Build history of the part. All positions in model axes, mm. Face numbers are marked on the shaded views. A direction names the side the tool comes from. Round coordinates to 2 decimals unless told otherwise and drop trailing zeros. Write each loop counter-clockwise with the first axis right and the second up, starting at its lowest first coordinate (ties: lowest second). Pieces come first, ordered by that corner, then holes. Notation, with made-up numbers: (19.5, -17) -> (32.5, -17) arc R13 ccw to (32.5, -10) -> close; hole circle Ø2 at (79.25, 52). An arc over 180 degrees is marked (long way). Answer in a Markdown table with one row per item.
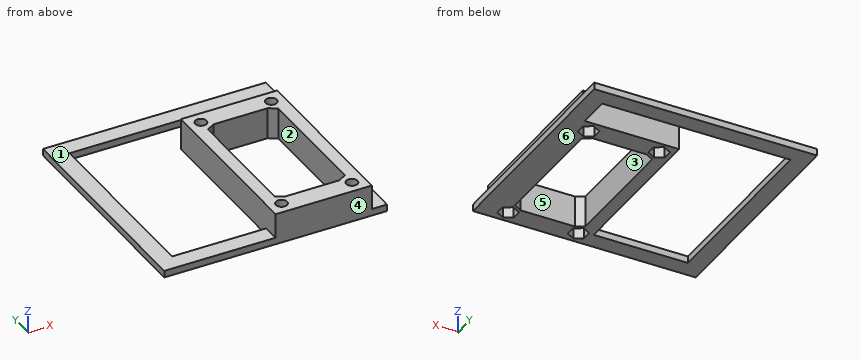
Autodesk Fusion 360 part; units mm, degrees
sketch "Sketch1" plane through (0, 0, 0) normal (0, 0, 1) x (1, 0, 0)
  line L0 (0, 0) -> (-65, 0)
  line L1 (-65, 0) -> (-65, 65)
  line L2 (-65, 65) -> (0, 65)
  line L3 (0, 65) -> (0, 0)
  line L4 (-32.5, 65) -> (-32.5, 0)
  line L5 (-28.75, 1) -> (-26.3684, 2.375)
  line L6 (-26.3684, 2.375) -> (-26.3684, 5.125)
  line L7 (-26.3684, 5.125) -> (-28.75, 6.5)
  line L8 (-28.75, 6.5) -> (-31.1316, 5.125)
  line L9 (-31.1316, 5.125) -> (-31.1316, 2.375)
  line L10 (-31.1316, 2.375) -> (-28.75, 1)
  line L11 (-28.75, 44.19) -> (-26.3684, 45.565)
  line L12 (-26.3684, 45.565) -> (-26.3684, 48.315)
  line L13 (-26.3684, 48.315) -> (-28.75, 49.69)
  line L14 (-28.75, 49.69) -> (-31.1316, 48.315)
  line L15 (-31.1316, 48.315) -> (-31.1316, 45.565)
  line L16 (-31.1316, 45.565) -> (-28.75, 44.19)
  line L17 (-28.75, 49.69) -> (-28.75, 50.69)
  line L18 (-28.75, 50.69) -> (-32.5, 50.69)
  line L19 (-28.75, 50.69) -> (0, 50.69)
  line L20 (-65, 0) -> (-60, 0)
  line L21 (-60, 0) -> (-60, 5)
  line L22 (-60, 5) -> (-65, 5)
  line L23 (-65, 5) -> (-65, 0)
  line L24 (-65, 65) -> (-60, 65)
  line L25 (-60, 65) -> (-60, 60)
  line L26 (-60, 60) -> (-65, 60)
  line L27 (-65, 60) -> (-65, 65)
  line L28 (0, 65) -> (-5, 65)
  line L29 (-5, 65) -> (-5, 60)
  line L30 (-5, 60) -> (0, 60)
  line L31 (0, 60) -> (0, 65)
  line L32 (-5, 60) -> (-60, 60)
  line L33 (-60, 60) -> (-60, 65)
  line L34 (-60, 65) -> (-5, 65)
  line L35 (-5, 65) -> (-5, 60)
  line L36 (-60, 60) -> (-65, 60)
  line L37 (-65, 60) -> (-65, 5)
  line L38 (-65, 5) -> (-60, 5)
  line L39 (-60, 5) -> (-60, 60)
  line L40 (-60, 0) -> (-32.5, 0)
  line L41 (-32.5, 0) -> (-32.5, 5)
  line L42 (-32.5, 5) -> (-60, 5)
  line L43 (-60, 5) -> (-60, 0)
  line L44 (-28.75, 6.5) -> (-28.75, 7.5)
  line L45 (-28.75, 7.5) -> (-26.3684, 6.125)
  line L46 (-28.75, 44.19) -> (-28.75, 43.19)
  line L47 (-3.75, 44.19) -> (-3.75, 43.19)
  line L48 (-26.3684, 44.565) -> (-28.75, 43.19)
  line L49 (-28.75, 7.5) -> (-28.75, 43.19)
  circle A0 centre (-28.75, 46.94) radius 1.65
  circle A1 centre (-28.75, 3.75) radius 1.65
  line L50 (-5, 60) -> (-5, 50.69)
  line L51 (-28.75, 46.94) -> (-8.2, 46.94)
  circle A2 centre (-8.2, 46.94) radius 1.65
  line L52 (-28.75, 3.75) -> (-8.2, 3.75)
  circle A3 centre (-8.2, 3.75) radius 1.65
  line L53 (-8.2, 1) -> (-5.8184, 2.375)
  line L54 (-5.8184, 2.375) -> (-5.8184, 5.125)
  line L55 (-5.8184, 5.125) -> (-8.2, 6.5)
  line L56 (-8.2, 6.5) -> (-10.5816, 5.125)
  line L57 (-10.5816, 5.125) -> (-10.5816, 2.375)
  line L58 (-10.5816, 2.375) -> (-8.2, 1)
  line L59 (-8.2, 44.19) -> (-5.8184, 45.565)
  line L60 (-5.8184, 45.565) -> (-5.8184, 48.315)
  line L61 (-5.8184, 48.315) -> (-8.2, 49.69)
  line L62 (-8.2, 49.69) -> (-10.5816, 48.315)
  line L63 (-10.5816, 48.315) -> (-10.5816, 45.565)
  line L64 (-10.5816, 45.565) -> (-8.2, 44.19)
  line L65 (-8.2, 44.19) -> (-8.2, 43.19)
  line L66 (-8.2, 43.19) -> (-10.5816, 44.565)
  line L67 (-10.5816, 44.565) -> (-26.3684, 44.565)
  line L68 (-8.2, 43.19) -> (-8.2, 7.5)
  line L69 (-8.2, 7.5) -> (-10.5816, 6.125)
  line L70 (-10.5816, 6.125) -> (-26.3684, 6.125)
  line L71 (-8.2, 25.345) -> (-4.45, 25.345)
  line L72 (-4.45, 25.345) -> (-4.45, 0)
  line L73 (-4.45, 25.345) -> (-4.45, 50.69)
  point P0 (-28.75, 3.75)
  point P1 (-28.75, 46.94)
  point P2 (-8.2, 3.75)
  point P3 (-8.2, 46.94)
  dimension "d1" = 65
  dimension "d2" = 65
  dimension "d10" = 43.19
  dimension "d12" = 2.75
  dimension "d14" = 1
  dimension "d15" = 1
  dimension "d17" = 3.3
  dimension "d20" = 3.3
  dimension "d27" = 20.55
  dimension "d28" = 3.3
  dimension "d29" = 20.55
  dimension "d30" = 3.3
  dimension "d31" = 2.75
  dimension "d32" = 1
  dimension "d33" = 3.75
extrude "Extrude4" add sketch "Sketch1" along normal blind 9.2 contours L53 L54 L55 L56 L57 L58 | L5 L6 L7 L8 L9 L10 | L0 L4 L14 L15 L16 L17 L18 L41 L45 L46 L49 L68 L69 L70 L71 L72 | L12 L13 L17 L19 L51 L59 L60 L61 L62 L63 L65 L68 L71 L73 | L11 L12 L46 L48 L51 L63 L64 L65 L66 L67 | L59 L60 L61 L62 L63 L64 | L11 L12 L13 L14 L15 L16
extrude "Extrude5" add sketch "Sketch1" along normal blind 2 contours L0 L3 L19 L72 L73 | L3 L19 L30 L50 | L0 L4 L21 L40 L41 L42 L43 | L2 L3 L28 L29 L30 L31 L35 | L0 L1 L20 L21 L22 L23 L38 L43 | L2 L4 L29 L32 L34 L35 | L1 L22 L26 L36 L37 L38 L39 | L2 L4 L25 L32 L33 L34 | L1 L2 L24 L25 L26 L27 L33 L36
extrude "Extrude6" cut sketch "Sketch1" along normal blind 6 contours L53 L54 L55 L56 L57 L58 | L5 L6 L7 L8 L9 L10 | L59 L60 L61 L62 L63 L64 | L11 L12 L13 L14 L15 L16
Q1. Wall check: line 1 (X direction, y = 28, z = 2.25); line 2 (X direction, y = 40.5, z = 1); line 3 (X direction, y = 56, z = 1.25). Give the ranges that are in metal, low to high. Write a range as [from, to].
A:
| item | result |
|---|---|
| line 1 | [-32.5, -28.75], [-8.2, -4.45] |
| line 2 | [-65, -60], [-32.5, -28.75], [-8.2, 0] |
| line 3 | [-65, -60], [-5, 0] |
Q2. Saw through at D-D on y = 46.94. Write the cut outline in (x, z).
A:
| item | result |
|---|---|
| outline | (-65, 0) -> (-60, 0) -> (-60, 2) -> (-65, 2) -> close; (-32.5, 0) -> (-31.13, 0) -> (-31.13, 6) -> (-30.4, 6) -> (-30.4, 9.2) -> (-32.5, 9.2) -> close; (-27.1, 6) -> (-26.37, 6) -> (-26.37, 0) -> (-10.58, 0) -> (-10.58, 6) -> (-9.85, 6) -> (-9.85, 9.2) -> (-27.1, 9.2) -> close; (-6.55, 6) -> (-5.82, 6) -> (-5.82, 0) -> (0, 0) -> (0, 2) -> (-4.45, 2) -> (-4.45, 9.2) -> (-6.55, 9.2) -> close |
Q3. Saw through at B-B on y = 12. Write the cut outline in (x, z).
A:
| item | result |
|---|---|
| outline | (-65, 0) -> (-60, 0) -> (-60, 2) -> (-65, 2) -> close; (-32.5, 0) -> (-28.75, 0) -> (-28.75, 9.2) -> (-32.5, 9.2) -> close; (-8.2, 0) -> (0, 0) -> (0, 2) -> (-4.45, 2) -> (-4.45, 9.2) -> (-8.2, 9.2) -> close |
Q4. Which spindle directions (+Z, -Z, +X, -X, +Y, -Y) get a long thin tool onto all of the face, cutting with end or side? Do the marked faces 5 and 6. Say none if no direction does.
A:
| item | result |
|---|---|
| face 5 | +Z, -Z |
| face 6 | -Z, +X, -X, +Y, -Y |
Q5. Saw through at A-A on x = -12. Write the cut outline in (y, z) (3 decimals).
A:
| item | result |
|---|---|
| outline | (0, 0) -> (6.125, 0) -> (6.125, 9.2) -> (0, 9.2) -> close; (44.565, 0) -> (50.69, 0) -> (50.69, 9.2) -> (44.565, 9.2) -> close; (60, 0) -> (65, 0) -> (65, 2) -> (60, 2) -> close |
Q6. Saw through at C-C on x = -43. Write the cut outline in (y, z).
A:
| item | result |
|---|---|
| outline | (0, 0) -> (5, 0) -> (5, 2) -> (0, 2) -> close; (60, 0) -> (65, 0) -> (65, 2) -> (60, 2) -> close |
Q7. Two-plate mould, pull along Y, no slides. Class the marked faces 1, 2, 3 and 4: released by +Y, released by -Y, zero draft, split by the parting line, or undercut.
A:
| item | result |
|---|---|
| face 1 | zero draft |
| face 2 | undercut |
| face 3 | undercut |
| face 4 | released by -Y |
Q8. Drop flat-ended pins along their axis: P1, Ø4, axis at x = -8.2, y = 3.75, coming from the -Z side; P2, Ø0.8, axis at y = 46.5, z = 4.5, coming from the -X side; P3, Ø2.5, axis at x = -8, y = 47, coming from the -Z side; P4, Ø3, axis at y = 3.5, z = 4.5, coming from the +X side. Give the stop position or say it passes through.
A:
| item | result |
|---|---|
| P1 | z = 6 |
| P2 | x = -32.5 |
| P3 | through |
| P4 | x = -4.45 |
